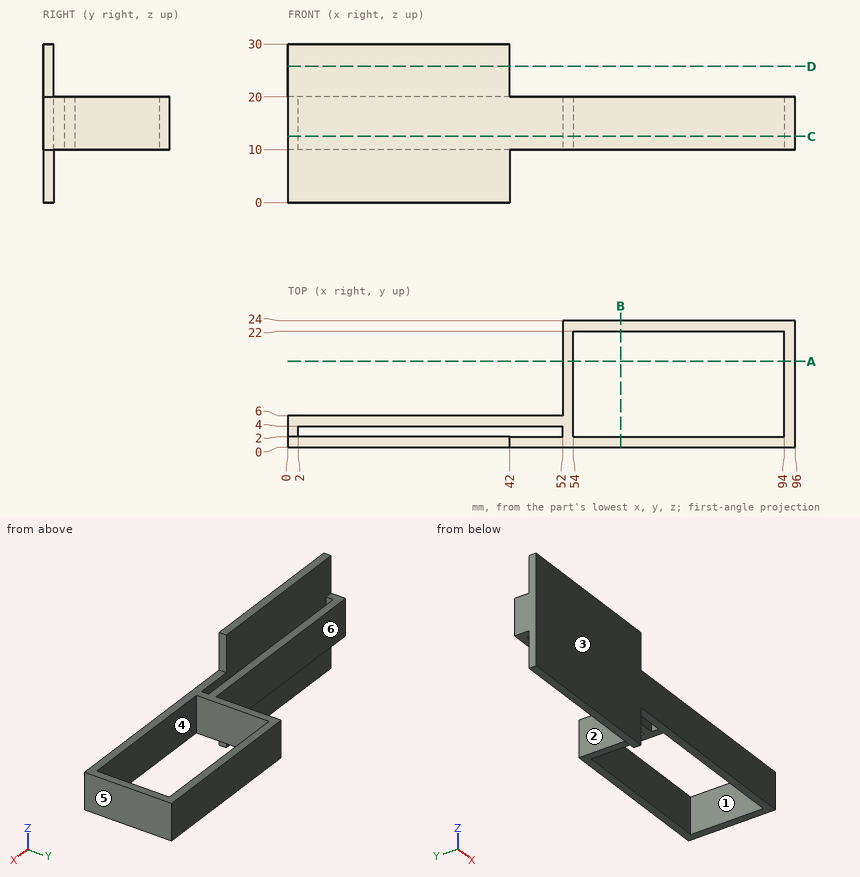
The figure shows three views and two pictorial views of one solid part (mm, origin at its lowest corner). Answer the questions. A direction names the side the tool comes from. Round coordinates to 2 decimals unless told otherwise and drop trailing zeros. Write each loop counter-clockwise with the first axis right and the second up, starting at its lowest first coordinate (ties: lowest second). Pieces come first, ordered by that corner, then holes. Notation, with made-up numbers: (5.25, 16) - (43.25, 16) arc R17 ccw to (43.25, 46) - close; hole circle Ø8 at (53.25, -36). An arc over 180 degrees is marked (long way). Use one line per item in the form item = value. Start each with the question number.
Item 1: A cutting plane is placed at B-B (x = 63). Write down the section's boundary in (y, z).
Item 2: Flat-ended cylindrical pins translate along their axes: pin 1 Ø8 at (y, z) = (16, 13.5) entering from -X; pin 2 Ø6 at (x, z) = (40, 14.5) entering from -Y; pin 3 Ø3 at (x, z) = (37, 16) entering from +Y; pin 4 Ø2 at (y, z) = (1.5, 4) entering from +X. Find the tip coordinate at first contact, or state that the pin passes through.
Item 3: A cutting plane is placed at D-D (z = 25.75). Write down the section's boundary in (x, y), plus the area to 3 significant figures.
Item 4: A tool of negligible diameter and unlimited length cuts with its end or side. For the marked faces 1, 2 and 3, from which of +Z, -Z, +X, -X, +Y, -Y can it reach the whole face along a straight path? Write none if from no direction.
Item 5: A cutting plane is placed at C-C (z = 12.5). Write down the section's boundary in (x, y).
Item 6: Determine the mould class of the marked faces 4, 5 and 6 for opening direction Y: +Y half, -Y half, draft (parallel to the pull), parting line (faces both ways), or undercut.
Item 7: Find the intervals of material crossed by line 1 (X direction, y = 12.5, z = 16); line 2 (X direction, y = 5, z = 11.75); line 3 (Y direction, x = 39, z = 22), in increasing order. Write a range as [from, to].
Item 8: A cutting plane is placed at A-A (y = 16.25). Write down the section's boundary in (x, z), plus the area to 3 significant figures.
The answers:
q1.outline = (0, 10) - (2, 10) - (2, 20) - (0, 20) - close; (22, 10) - (24, 10) - (24, 20) - (22, 20) - close
q2.pin_1 = 52
q2.pin_2 = 0
q2.pin_3 = 6
q2.pin_4 = 42
q3.outline = (0, 0) - (42, 0) - (42, 2) - (0, 2) - close
q3.area = 84.0 mm^2
q4.face_1 = +Z, -Z
q4.face_2 = +Z, -Z, -X, +Y
q4.face_3 = +Z, -Z, +X, -X, -Y
q5.outline = (0, 0) - (96, 0) - (96, 24) - (52, 24) - (52, 6) - (0, 6) - close; hole (2, 2) - (52, 2) - (52, 4) - (2, 4) - close; hole (54, 2) - (94, 2) - (94, 22) - (54, 22) - close
q6.face_4 = undercut
q6.face_5 = draft
q6.face_6 = +Y half
q7.line_1 = [52, 54], [94, 96]
q7.line_2 = [0, 54], [94, 96]
q7.line_3 = [0, 2]
q8.outline = (52, 10) - (54, 10) - (54, 20) - (52, 20) - close; (94, 10) - (96, 10) - (96, 20) - (94, 20) - close
q8.area = 40.0 mm^2
